from build123d import *

# Parameters (mm, degrees)
SKETCH1_R           = 3
SKETCH1_R_2         = 4.5
SKETCH1_R_3         = 1.6
BOSS_EXTRUDE3_DEPTH = 1.6
SKETCH2_R           = 1.6
SKETCH2_R_2         = 3
SKETCH2_R_3         = 4.5
BOSS_EXTRUDE4_DEPTH = 1.5
SKETCH3_R           = 63.206562555
CUT_EXTRUDE1_DEPTH  = 1.6
SKETCH4_R           = 3
SKETCH4_R_2         = 1.6
BOSS_EXTRUDE5_DEPTH = 1.5


with BuildPart() as part:
    # Sketch1 → Boss-Extrude3 (new body)
    with BuildSketch(Plane.XY):
        with BuildLine():
            Line((12.073070054, 14.639688463), (24.958502044, 12.880515151))
            ThreePointArc((24.958502044, 12.880515151), (36.2, 0), (24.958502044, -12.880515151))
            Line((24.958502044, -12.880515151), (12.073070054, -14.639688463))
            ThreePointArc((12.073070054, -14.639688463), (11.870633815, -14.660360595), (11.66726189, -14.66726189))
            Line((11.66726189, -14.66726189), (0, -14.66726189))
            ThreePointArc((0, -14.66726189), (-0.888679088, -14.53261518), (-1.697586366, -14.140761542))
            Line((-1.697586366, -14.140761542), (-18.697586366, -2.473499652))
            ThreePointArc((-18.697586366, -2.473499652), (-19.891071988, -0.801063519), (-19.728500117, 1.247111507))
            Line((-19.728500117, 1.247111507), (-14.395762007, 12.914373397))
            ThreePointArc((-14.395762007, 12.914373397), (-13.288783625, 14.191279968), (-11.66726189, 14.66726189))
            Line((-11.66726189, 14.66726189), (11.66726189, 14.66726189))
            ThreePointArc((11.66726189, 14.66726189), (11.870633815, 14.660360595), (12.073070054, 14.639688463))
        make_face()
        Circle(SKETCH1_R, mode=Mode.SUBTRACT)
        with Locations((23.2, 0)):
            Circle(SKETCH1_R_2, mode=Mode.SUBTRACT)
        with Locations((8.6, 0)):
            Circle(SKETCH1_R, mode=Mode.SUBTRACT)
        with Locations((-17, 0)):
            Circle(SKETCH1_R_3, mode=Mode.SUBTRACT)
        with Locations((0, -11.66726189)):
            Circle(SKETCH1_R_3, mode=Mode.SUBTRACT)
        with Locations((11.66726189, -11.66726189)):
            Circle(SKETCH1_R_3, mode=Mode.SUBTRACT)
        with Locations((-11.66726189, 11.66726189)):
            Circle(SKETCH1_R_3, mode=Mode.SUBTRACT)
        with Locations((0, 11.66726189)):
            Circle(SKETCH1_R_3, mode=Mode.SUBTRACT)
        with Locations((11.66726189, 11.66726189)):
            Circle(SKETCH1_R_3, mode=Mode.SUBTRACT)
    extrude(amount=BOSS_EXTRUDE3_DEPTH)

    # Sketch2 → Boss-Extrude4 (add)
    with BuildSketch(Plane.XY.offset(1.6)):
        with BuildLine():
            Line((12.073070054, 14.639688463), (24.958502044, 12.880515151))
            ThreePointArc((24.958502044, 12.880515151), (36.2, 0), (24.958502044, -12.880515151))
            Line((24.958502044, -12.880515151), (12.073070054, -14.639688463))
            ThreePointArc((12.073070054, -14.639688463), (10.884137398, -14.56324463), (9.81871257, -14.030070687))
            Line((9.81871257, -14.030070687), (-3.080915533, -3.938014662))
            ThreePointArc((-3.080915533, -3.938014662), (-5, 0), (-3.080915533, 3.938014662))
            Line((-3.080915533, 3.938014662), (9.81871257, 14.030070687))
            ThreePointArc((9.81871257, 14.030070687), (10.884137398, 14.56324463), (12.073070054, 14.639688463))
        make_face()
        with Locations((11.66726189, 11.66726189)):
            Circle(SKETCH2_R, mode=Mode.SUBTRACT)
        Circle(SKETCH2_R_2, mode=Mode.SUBTRACT)
        with Locations((8.6, 0)):
            Circle(SKETCH2_R_2, mode=Mode.SUBTRACT)
        with Locations((23.2, 0)):
            Circle(SKETCH2_R_3, mode=Mode.SUBTRACT)
        with Locations((11.66726189, -11.66726189)):
            Circle(SKETCH2_R, mode=Mode.SUBTRACT)
    extrude(amount=BOSS_EXTRUDE4_DEPTH)

    # Sketch3 → Cut-Extrude1 (cut)
    with BuildSketch(Plane(origin=(0, 0, 0), x_dir=(-1, 0, 0), z_dir=(0, 0, -1))):
        Circle(SKETCH3_R)
    extrude(amount=-CUT_EXTRUDE1_DEPTH, mode=Mode.SUBTRACT)

    # Sketch4 → Boss-Extrude5 (add)
    with BuildSketch(Plane.XY.offset(3.1)):
        with BuildLine():
            Line((-3.602159399, 6.00203696), (10.12347929, 14.239563444))
            ThreePointArc((10.12347929, 14.239563444), (13.145208472, 14.277946455), (14.66726189, 11.66726189))
            Line((14.66726189, 11.66726189), (14.66726189, -11.66726189))
            ThreePointArc((14.66726189, -11.66726189), (13.145208472, -14.277946455), (10.12347929, -14.239563444))
            Line((10.12347929, -14.239563444), (-3.602159399, -6.00203696))
            ThreePointArc((-3.602159399, -6.00203696), (-7, 0), (-3.602159399, 6.00203696))
        make_face()
        Circle(SKETCH4_R, mode=Mode.SUBTRACT)
        with Locations((8.6, 0)):
            Circle(SKETCH4_R, mode=Mode.SUBTRACT)
        with Locations((11.66726189, 11.66726189)):
            Circle(SKETCH4_R_2, mode=Mode.SUBTRACT)
        with Locations((11.66726189, -11.66726189)):
            Circle(SKETCH4_R_2, mode=Mode.SUBTRACT)
    extrude(amount=-BOSS_EXTRUDE5_DEPTH)


solid = part.part
Here's how the part is built. I have some questions about the finished solid (model axes, mm). Give positions to 0.01 mm unless a question says otherwise; leave off trailing zeros. Loops run counter-clockwise (first coordinate to the right, second up) from the corner with the lowest first, then second, coordinate; pieces in that order, holes last. Notation, with made-up numbers: (-38, 68.5) -> (0, 68.5) arc R17 cw to (0, 88.5) -> close; hole circle Ø8 at (-10.75, -39). An arc over 180 degrees is marked (long way). Answer as a JSON object with one key per item and string values. Group by question number.
Item 1: Imagine slicing it at D-D on z = 2.2. Write out the boundary of the cut face in (x, y).
Item 2: Imagine slicing it at A-A on y = 0. Write out the boundary of the cut face in (x, z), then the cut area to 3 significant figures.
Item 3: I need wall thicknesses on L1, parallel to X at y = 0.5, z = 3; L2, parallel to X at y = -2.25, z = 2.9; L3, parallel to Y at x = 7.5, z = 1.85. Which ranges of each line are inside material? Lowest first, please.
Item 4: Imagine slicing it at C-C on y = -12.25. Write out the boundary of the cut face in (x, z), then the cut area to 3 significant figures.
Item 5: Thinking about a two-plate mould opening in X: for faces 1 (the cylindrical face through (-3, 0, 2)), 2 (the flat face through (3.36, -10.18, 2.36)), 3 (the cylindrical face through (5.6, 0.1, 2.3)), 4 (the flat face through (18.606, -13.748, 2.34)), which applies, pulls with the +X half, pulls with the -X half, needs draft (parallel to the pull), parting line crosses it, or undercut?
Item 6: Imagine slicing it at B-B on x = 7.5. Write out the boundary of the cut face in (y, z).
Answer list:
{
 "1": {"outline": "(-3.6, -6) -> (10.12, -14.24) arc R3 ccw to (12.07, -14.64) -> (24.96, -12.88) arc R13 ccw to (24.96, 12.88) -> (12.07, 14.64) arc R3 ccw to (10.12, 14.24) -> (-3.6, 6) arc R7 ccw to start; hole circle Ø6 at (0, 0); hole circle Ø6 at (8.6, 0); hole circle Ø3.2 at (11.67, -11.67); hole circle Ø3.2 at (11.67, 11.67); hole circle Ø9 at (23.2, 0)"},
 "2": {"outline": "(-7, 1.6) -> (-3, 1.6) -> (-3, 3.1) -> (-7, 3.1) -> close; (3, 1.6) -> (5.6, 1.6) -> (5.6, 3.1) -> (3, 3.1) -> close; (11.6, 1.6) -> (18.7, 1.6) -> (18.7, 3.1) -> (11.6, 3.1) -> close; (27.7, 1.6) -> (36.2, 1.6) -> (36.2, 3.1) -> (27.7, 3.1) -> close", "area": "33.3 mm2"},
 "3": {"L1": "x = -6.98 to -2.96, 2.96 to 5.64, 11.56 to 18.73, 27.67 to 36.19", "L2": "x = -6.63 to -1.98, 1.98 to 6.62, 10.58 to 19.3, 27.1 to 36", "L3": "y = -12.67 to -2.79, 2.79 to 12.67"},
 "4": {"outline": "(6.81, 1.6) -> (10.18, 1.6) -> (10.18, 3.1) -> (6.81, 3.1) -> close; (13.16, 1.6) -> (27.55, 1.6) -> (27.55, 3.1) -> (13.16, 3.1) -> close", "area": "26.6 mm2"},
 "5": {"face 1": "undercut", "face 2": "pulls with the -X half", "face 3": "undercut", "face 4": "pulls with the +X half"},
 "6": {"outline": "(-12.67, 1.6) -> (-2.79, 1.6) -> (-2.79, 3.1) -> (-12.67, 3.1) -> close; (2.79, 1.6) -> (12.67, 1.6) -> (12.67, 3.1) -> (2.79, 3.1) -> close"}
}
